Study the drawing (mm; zero at the part's minimum x, y, z) and answer. A direction names the side the tool comes from. Round coordinates to 2 decimals unless told otherwise and drop trailing zeros. Loops run counter-clockwise (first coordinate to the right, second up) from the corner with the lowest first, then second, coordinate; pieces in that order, holes last. Notation, with made-up numbers: (61.5, 83.5) - (72.5, 83.5) arc R35 cw to (72.5, 117.5) - close; hole circle Ø8 at (-32.75, 51.5). An arc over 180 degrees is marked (long way). Use CSV: the item, a comma, the result in double quotes. Start each with the question number.
1. Determine the mould class of the marked faces 4, 5, 6 and 7 for opening direction Y: +Y half, -Y half, draft (parallel to the pull), parting line (faces both ways), or undercut.
2. Find section A-A (y = 32). State how many separate pieces and enclosed holes the cut face has, and give its area (3 significant figures).
3. Given pin 1 Ø20.5 at (y, z) = (38.31, 88.8) entering from +X; pin 2 Ø2 at (y, z) = (15.5, 42.5) entering from -X; pin 3 Ø8 at (y, z) = (47.5, 60.5) entering from -X; pin 4 Ø6 at (y, z) = (50, 44) entering from +X, each flat-ended and moving along its own axis, determine where each tip first touches the part or whether it passes through.
4. Find section C-C (y = 91). Give the vertices of the cut face in (x, z).
5. A tool of negligible diameter and unlimited length cuts with its end or side. For the marked faces 1, 2 and 3, from which of +Z, -Z, +X, -X, +Y, -Y can it reach the whole face along a straight path? Write none if from no direction.
6. Find section D-D (x = 116.5). Give the vertices of the cut face in (y, z), and give its area (3 significant figures).
7. Consider line 1 along Y through (x, z) = (23, 111.5); line 2 along Z through (x, y) = (144, 77) (1 decimal); line 3 along Z through (x, y) = (62, 114). Determine where each line is inside the solid, lowest interval first.
8. Find section B-B (z = 86). Give the vertices of the cut face in (x, y) (1 decimal), and give its area (3 significant figures).
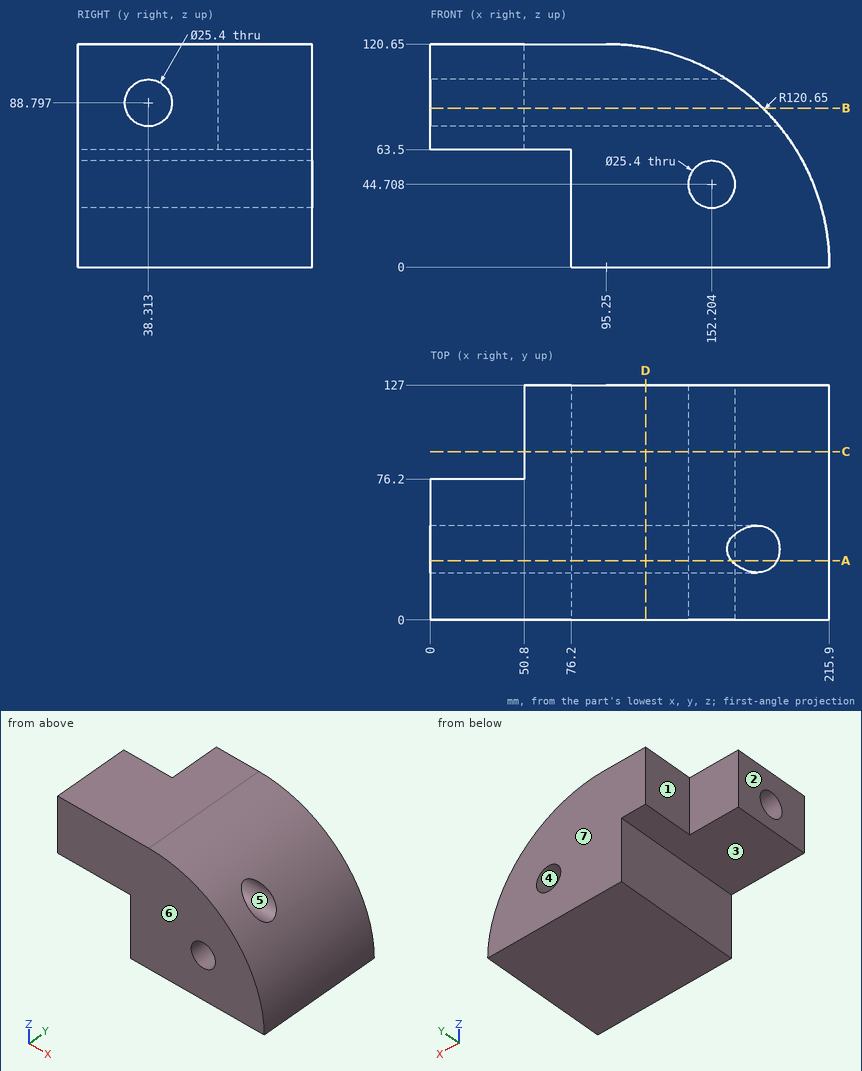
Filled sheet:
1,face 4,"draft"
1,face 5,"undercut"
1,face 6,"-Y half"
1,face 7,"+Y half"
2,separate pieces,"2"
2,enclosed holes,"1"
2,area,"13,700 mm²"
3,pin 1,"passes through"
3,pin 2,"stops at x = 76.2"
3,pin 3,"stops at x = 0"
3,pin 4,"stops at x = 208.72"
4,outline,"(50.8, 63.5) - (76.2, 63.5) - (76.2, 0) - (215.9, 0) arc R120.65 ccw to (95.25, 120.65) - (50.8, 120.65) - close; hole circle Ø25.4 at (152.2, 44.71)"
5,face 1,"+Z, -Z, -X, +Y"
5,face 2,"+Z, -Z, -X, +Y, -Y"
5,face 3,"-Z, -X, +Y, -Y"
6,outline,"(0, 0) - (127, 0) - (127, 118.76) - (0, 118.76) - close; hole circle Ø25.4 at (38.31, 88.8)"
6,area,"14,600 mm²"
7,line 1,"y = 0 to 76.2"
7,line 2,"z = 0 to 35, 54.4 to 110.4"
7,line 3,"z = 63.5 to 120.65"
8,outline,"(0, 0) - (179.9, 0) - (179.9, 25.9) - (0, 25.9) - close; (0, 50.7) - (179.9, 50.7) - (179.9, 127) - (50.8, 127) - (50.8, 76.2) - (0, 76.2) - close"
8,area,"15,800 mm²"
